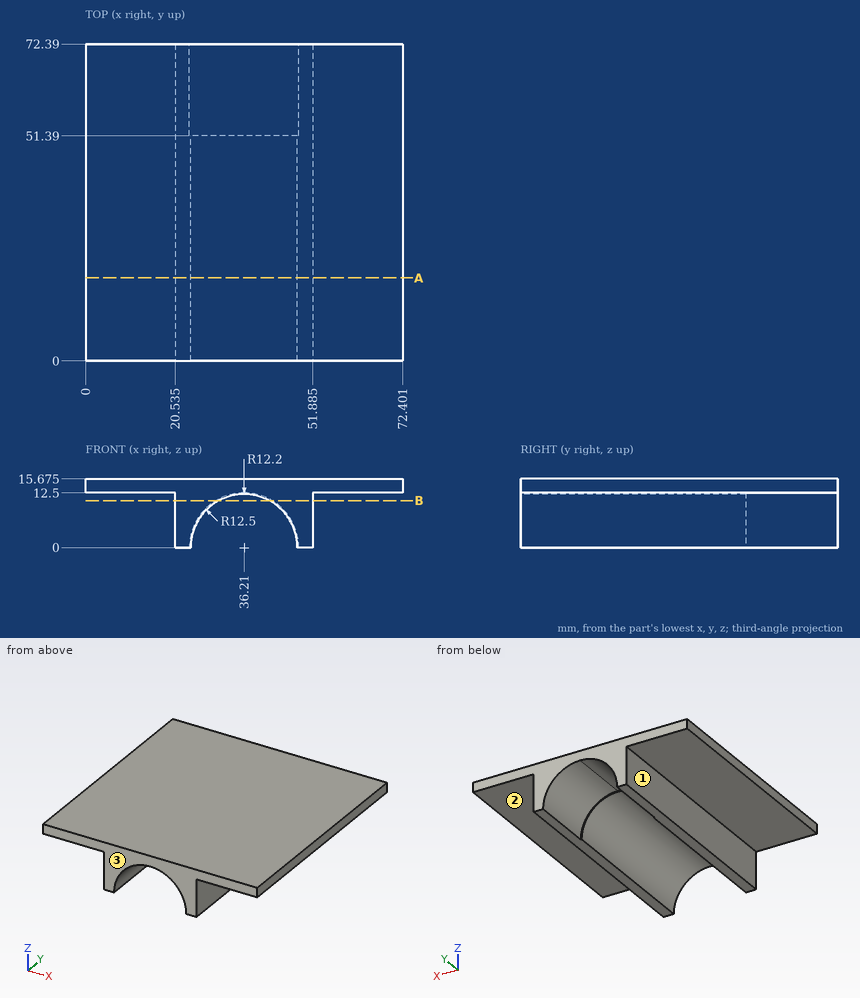
Print and shaded views of the part. All mm, measured from the part's lowest x, y and z. A direction names the side the tool comes from. Give positions to 0.01 mm unless a question says otherwise; leave off trailing zeros. Loops run counter-clockwise (first coordinate to the right, second up) from the corner with the lowest first, then second, coordinate; pieces in that order, holes last. Notation, with made-up numbers: (68.25, -26.5) -> (103.25, -26.5) arc R27 ccw to (103.25, -3.5) -> close; hole circle Ø10 at (79, 6.25). An arc over 180 degrees is marked (long way). Use CSV: the item, a comma, the result in double quotes. Start each with the question number.
1) Wall check: line 1 (Z direction, x = 6.5, y = 3.5) (1 decimal); line 2 (X direction, y = 3.5, z = 6) (1 decimal); line 3 (X direction, y = 57, z = 9.75) (1 decimal). Give the ranges that are in metal, low to high.
2) Tool access for the marked faces 1, 2 and 3: list every direction of +Z, -Z, +X, -X, +Y, -Y with a clear straight run to the whole face (end or side of a thin tool).
3) Slice it at B-B on z = 10.75. Give the cut face in (x, y) (1 decimal), plus the area to 3 significant figures.
4) Slice it at A-A on y = 19. Give the cut face in (x, z) (1 decimal), plus the area to 3 significant figures.
5) Flat gauge pins, fed straight in: pin 1 Ø6 at (x, y) = (63, 51.5) entering from -Z; pin 2 Ø4 at (y, z) = (49.5, 4.5) entering from +X (3 decimals); pin 3 Ø6 at (y, z) = (39, 3.5) entering from -X (3 decimals). Where does each tip first touch, or does it go through?
Computed values:
1,line 1,"z = 12.5 to 15.7"
1,line 2,"x = 20.5 to 25.6, 46.8 to 51.9"
1,line 3,"x = 20.5 to 28.4, 44 to 51.9"
2,face 1,"-Z, -X, +Y, -Y"
2,face 2,"-Z, +X, +Y, -Y"
2,face 3,"+Z, -Z, +X, -X, -Y"
3,outline,"(20.5, 0) -> (30.4, 0) -> (30.4, 51.4) -> (29.8, 51.4) -> (29.8, 72.4) -> (20.5, 72.4) -> close; (42, 0) -> (51.9, 0) -> (51.9, 72.4) -> (42.6, 72.4) -> (42.6, 51.4) -> (42, 51.4) -> close"
3,area,"1,410 mm^2"
4,outline,"(0, 12.5) -> (20.5, 12.5) -> (20.5, 0) -> (24, 0) arc R12.2 cw to (48.4, 0) -> (51.9, 0) -> (51.9, 12.5) -> (72.4, 12.5) -> (72.4, 15.7) -> (0, 15.7) -> close"
4,area,"388 mm^2"
5,pin 1,"stops at z = 12.5"
5,pin 2,"stops at x = 51.885"
5,pin 3,"stops at x = 20.535"
